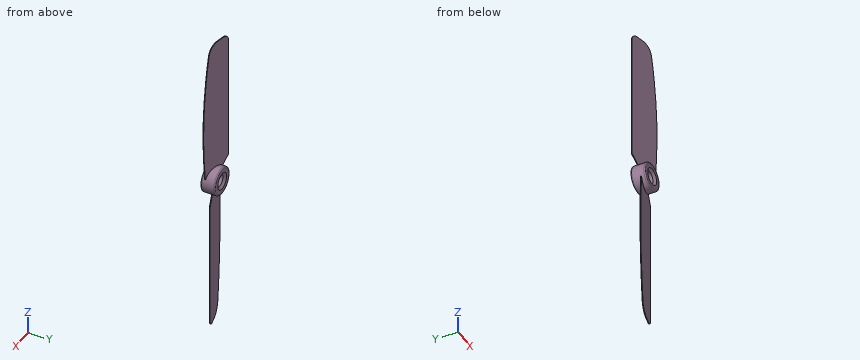
```python
from build123d import *

# Parameters (mm, degrees)
SKETCH1_R           = 5.75
BOSS_EXTRUDE1_DEPTH = 3
BOSS_EXTRUDE2_DEPTH = 0.15
CIRPATTERN1_COUNT   = 2
SKETCH4_R           = 2.5
CUT_EXTRUDE1_DEPTH  = 65.203765671
FILLET1_R           = 0.5
CHAMFER1_SIZE       = 1
CHAMFER2_SIZE       = 1


with BuildPart() as part:
    # Sketch1 → Boss-Extrude1 (new, symmetric)
    with BuildSketch(Plane(origin=(0, 0, 0), x_dir=(1, 0, 0), z_dir=(0, 1, 0))):
        with Locations(Location((0, 0, 0), (0, 0, 270))):
            Circle(SKETCH1_R)
    extrude(amount=BOSS_EXTRUDE1_DEPTH, both=True)

    # Sketch3 → Boss-Extrude2 (add, symmetric)
    with BuildSketch(Plane(origin=(0, 0, 0), x_dir=(0.9743700647852352, -0.22495105434386534, 0), z_dir=(-0.22495105434386534, -0.9743700647852352, 0))):
        with BuildLine():
            Line((-3.652357561, 3.652357561), (-7.49829587, 7.49829587))
            Line((-7.49829587, 7.49829587), (-7.49829587, 60.5))
            ThreePointArc((-7.49829587, 60.5), (-6.619616214, 62.621320344), (-4.49829587, 63.5))
            Line((-4.49829587, 63.5), (-1.464719741, 63.5))
            ThreePointArc((-1.464719741, 63.5), (1.755916544, 62.324591732), (3.462327822, 59.351000768))
            add(Edge.make_bspline(
                [(5.579389338, 2.779553643), (7.404721725, 21.734683746), (6.697564401, 40.619919544), (3.462327822, 59.351000768)],
                knots=[0, 0, 0, 0, 0.931210361, 0.931210361, 0.931210361, 0.931210361], degree=3))
            add(Edge.make_bspline(
                [(5.579389338, 2.779553643), (1.589885299, 10.194259474), (-3.652357561, 3.652357561)],
                knots=[5.216924211, 5.216924211, 5.216924211, 7.165723747, 7.165723747, 7.165723747], degree=2, weights=[1, 0.561664766, 1]))
        make_face()
    boss_extrude2 = extrude(amount=BOSS_EXTRUDE2_DEPTH, both=True)

    # CirPattern1: Boss-Extrude2 ×2 about axis
    cirpattern1_axis = Axis((0, 3, 0), (0, -1, 0))
    for i in range(1, CIRPATTERN1_COUNT):
        add(boss_extrude2.rotate(cirpattern1_axis, i * 360 / CIRPATTERN1_COUNT))

    # Sketch4 → Cut-Extrude1 (cut, through all)
    with BuildSketch(Plane.XZ.offset(3)):
        with Locations(Location((0, 0, 0), (0, 0, 270))):
            Circle(SKETCH4_R)
    extrude(amount=-CUT_EXTRUDE1_DEPTH, mode=Mode.SUBTRACT)

    # Fillet1
    fillet1_edges = [part.edges().sort_by_distance(p)[0] for p in [
        (0, -3, -5.75),
        (0, 3, -5.75),
    ]]
    fillet(fillet1_edges, radius=FILLET1_R)

    # Chamfer1
    chamfer1_edges = [part.edges().sort_by_distance(p)[0] for p in [
        (0, -3, 2.5),
    ]]
    chamfer(chamfer1_edges, length=CHAMFER1_SIZE)

    # Chamfer2
    chamfer2_edges = [part.edges().sort_by_distance(p)[0] for p in [
        (0, 3, 2.5),
    ]]
    chamfer(chamfer2_edges, length=CHAMFER2_SIZE)


solid = part.part
```
Geometry check sheet. Reference: the model listing, model coordinates, mm. Coordinates: 2 decimals unless noted, no trailing zeros. Write each loop counter-clockwise with the first axis right and the second up, starting at its lowest first coordinate (ties: lowest second). Pieces come first, ordered by that corner, then holes. Notation, with made-up numbers: M -17.5,85.5 L 16.5,85.5 A17 ccw 16.5,94.5 Z; hole C 2.5,52.5 d6. An arc over 180 degrees is marked long. One line per item, written item: value. Start each with the question number.
(1) Depth check by flat-ended pin: pin 1 (1 mm diameter, centred on x = -3.5, z = 39.5, fed in from +Y); pin 2 (1 mm diameter, centred on x = 1, y = 2, fed in from +Z); pin 3 (1.5 mm diameter, centred on x = -3, z = -47, fed in from +Y); pin 4 (8 mm diameter, centred on x = 0, z = 0, fed in from +Y). Enter the tip coordinate at first touch or a pass-through.
(2) Sectioned sample at A-A, the plane z = 0. Enter the section's corners in (x, y), and give its area (3 significant figures).
(3) Scan lines: line 1 along X through (y, z) = (0, 0); line 2 along Y through (x, z) = (1.5, -31); line 3 along Z through (x, y) = (1.5, 0.25). Record each from-to range of solid material in increasing order. Write a range as [from, to].
Filled sheet:
1. pin 1: y = 1.08
1. pin 2: z = 5.73
1. pin 3: y = -0.37
1. pin 4: y = 3
2. outline: M -5.75,-2.5 A0.5 ccw -5.25,-3 L -3.5,-3 L -2.5,-2 L -2.5,2 L -3.5,3 L -5.25,3 A0.5 ccw -5.75,2.5 Z; M 2.5,-2 L 3.5,-3 L 5.25,-3 A0.5 ccw 5.75,-2.5 L 5.75,2.5 A0.5 ccw 5.25,3 L 3.5,3 L 2.5,2 Z
2. area: 36.8 mm²
3. line 1: [-5.75, -2.5], [2.5, 5.75]
3. line 2: [0.19, 0.5]
3. line 3: [-63.5, -2], [2, 5.55]
